```python
from build123d import *

# Parameters (mm, degrees)
SKETCH1_R                  = 1.5
BOSS_EXTRUDE1_DEPTH        = 2.54
BOSS_EXTRUDE3_DEPTH        = 15
SKETCH5_R                  = 1.5
CUT_EXTRUDE1_DEPTH         = 12.7
CHAMFER1_SIZE              = 2.54
CHAMFER1_SIZE_2            = 4.399409051
CUT_EXTRUDE5_DEPTH         = 36.401142437
CHAMFER1_OF_MIRROR1_SIZE   = 4.399409051
CHAMFER1_OF_MIRROR1_SIZE_2 = 2.54


with BuildPart() as part:
    # Sketch1 → Boss-Extrude1 (new body)
    with BuildSketch(Plane(origin=(0, 0, 0), x_dir=(1, 0, 0), z_dir=(0, 1, 0))):
        with BuildLine():
            Line((-2.46, 6.35), (20.4, 6.35))
            ThreePointArc((20.4, 6.35), (22.196051224, 5.606051224), (22.94, 3.81))
            Line((22.94, 3.81), (22.94, -3.81))
            ThreePointArc((22.94, -3.81), (22.196051224, -5.606051224), (20.4, -6.35))
            Line((20.4, -6.35), (-2.46, -6.35))
            ThreePointArc((-2.46, -6.35), (-4.256051224, -5.606051224), (-5, -3.81))
            Line((-5, -3.81), (-5, 3.81))
            ThreePointArc((-5, 3.81), (-4.256051224, 5.606051224), (-2.46, 6.35))
        make_face()
        with Locations(Location((-1.19, -2.88414655, 0), (0, 0, 270))):
            Circle(SKETCH1_R, mode=Mode.SUBTRACT)
        with Locations(Location((8.81, -2.88414655, 0), (0, 0, 270))):
            Circle(SKETCH1_R, mode=Mode.SUBTRACT)
        with Locations(Location((18.81, -2.88414655, 0), (0, 0, 270))):
            Circle(SKETCH1_R, mode=Mode.SUBTRACT)
    boss_extrude1 = extrude(amount=BOSS_EXTRUDE1_DEPTH)

    # Sketch3 → Boss-Extrude3 (add)
    with BuildSketch(Plane(origin=(0, 2.54, 0), x_dir=(1, 0, 0), z_dir=(0, 1, 0))):
        with BuildLine():
            Line((-5, 2.54), (22.94, 2.54))
            Line((22.94, 2.54), (22.94, 3.81))
            Line((22.94, 3.81), (22.94, 19.207931679))
            ThreePointArc((22.94, 19.207931679), (22.305, 20.307783942), (21.035, 20.307783942))
            Line((21.035, 20.307783942), (-3.73, 6.009704526))
            ThreePointArc((-3.73, 6.009704526), (-4.659704526, 5.08), (-5, 3.81))
            Line((-5, 3.81), (-5, 2.54))
        make_face()
    boss_extrude3 = extrude(amount=BOSS_EXTRUDE3_DEPTH)

    # Sketch5 → Cut-Extrude1 (cut)
    with BuildSketch(Plane(origin=(-5.860422493, 0, -4.779704526), x_dir=(0.8660254037844379, 0, -0.5000000000000014), z_dir=(0.5000000000000013, 0, 0.8660254037844378))):
        with Locations(Location((6.758079416, 6.35, 0), (0, 0, 180))):
            Circle(SKETCH5_R)
        with Locations(Location((26.758079416, 6.35, 0), (0, 0, 180))):
            Circle(SKETCH5_R)
    cut_extrude1 = extrude(amount=CUT_EXTRUDE1_DEPTH, mode=Mode.SUBTRACT)

    # Chamfer1
    # the kernel refuses this chamfer: 4.399409051, 2.54 mm, written as the material it adds along each edge
    with BuildSketch(Plane(origin=(-5, 2.54, -2.54), x_dir=(0, -0.057893862402671366, 0.9983227437537925), z_dir=(1, 0, 0))) as chamfer1_piece_1_section:
        Polygon((CHAMFER1_SIZE * 0.998322743754, -CHAMFER1_SIZE * 0.0578938624027), (-CHAMFER1_SIZE_2 * 0.0578938624056, -CHAMFER1_SIZE_2 * 0.998322743805), (0, 0), align=None)
    chamfer1_piece_1 = extrude(amount=27.94, mode=Mode.PRIVATE)
    chamfer1_piece_1 = chamfer1_piece_1 - Plane(origin=(5.060500306, 6.35, 0.619729795), x_dir=(-0.8660254037844379, 0, 0.5000000000000014), z_dir=(-0.5000000000000014, 0, -0.8660254037844379)) * Cylinder(1.5, 74, mode=Mode.PRIVATE)
    add(chamfer1_piece_1)

    # Sketch11 → Cut-Extrude5 (cut, symmetric)
    with BuildSketch(Plane(origin=(0, 17.54, 0), x_dir=(1, 0, 0), z_dir=(0, 1, 0))):
        Polygon((3.153238686, 9.983744234), (4.423238686, 7.784039708), (15.421761314, 14.134039708), (14.151761314, 16.333744234), align=None)
    cut_extrude5 = extrude(amount=CUT_EXTRUDE5_DEPTH, both=True, mode=Mode.SUBTRACT)

    # Mirror1: Boss-Extrude1, Boss-Extrude3, Cut-Extrude1, Cut-Extrude5 across plane
    add(boss_extrude1.mirror(Plane.XY.offset(2.88414655)))
    add(boss_extrude3.mirror(Plane.XY.offset(2.88414655)))
    add(cut_extrude1.mirror(Plane.XY.offset(2.88414655)), mode=Mode.SUBTRACT)
    add(cut_extrude5.mirror(Plane.XY.offset(2.88414655)), mode=Mode.SUBTRACT)

    # Chamfer1 of Mirror1
    # the kernel refuses this chamfer: 4.399409051, 2.54 mm, written as the material it adds along each edge
    with BuildSketch(Plane(origin=(-5, 2.54, 8.308293101), x_dir=(0, 0.9998132206222079, 0.019326765612700737), z_dir=(1, 0, 0))) as chamfer1_of_mirror1_piece_1_section:
        Polygon((CHAMFER1_OF_MIRROR1_SIZE * 0.999813220673, -CHAMFER1_OF_MIRROR1_SIZE * 0.0193267656137), (-CHAMFER1_OF_MIRROR1_SIZE_2 * 0.0193267656127, -CHAMFER1_OF_MIRROR1_SIZE_2 * 0.999813220622), (0, 0), align=None)
    chamfer1_of_mirror1_piece_1 = extrude(amount=27.94, mode=Mode.PRIVATE)
    chamfer1_of_mirror1_piece_1 = chamfer1_of_mirror1_piece_1 - Plane(origin=(5.060500238, 6.35, 5.148563423), x_dir=(-0.8660254037844379, 0, -0.5000000000000014), z_dir=(-0.5000000000000014, 0, 0.8660254037844379)) * Cylinder(1.5, 74, mode=Mode.PRIVATE)
    add(chamfer1_of_mirror1_piece_1)


solid = part.part
```
Geometry: final body of the model. Coordinates: model frame, mm. A direction names the side the tool comes from. Round coordinates to 2 decimals unless told otherwise and drop trailing zeros. Order: outer loops, then holes, each group sorted by start corner. A loop starts at its lowest first (then second) coordinate and runs counter-clockwise, first axis right, second up. Notation, with made-up numbers: (-1, 76.5) -> (14, 76.5) arc R22 cw to (14, 98.5) -> close; hole circle Ø4 at (19.5, 68). An arc over 180 degrees is marked (long way). Use one line per item in the form item = value.
(1) First-contact query: pin 1 Ø5 at (x, z) = (13.5, 18.5) entering from -Y; pin 2 Ø2 at (x, y) = (11.5, 14) entering from -Z; pin 3 Ø6 at (x, y) = (0.5, 8.5) entering from -Z. Flat tips, straight axial feed; report the tip coordinate or a pass-through.
Results list:
pin_1 = 2.54
pin_2 = -12.45
pin_3 = -9.98
(2) Section B-B on x = 8.81. Return loops of the section in (y, z), and give its area (3 significant figures).
Results list:
outline = (0, -6.35) -> (2.54, -6.35) -> (2.54, -10.32) -> (17.54, -10.32) -> (17.54, -2.54) -> (6.94, -2.54) -> (2.54, 0) -> (2.54, 1.38) -> (0, 1.38) -> close; (0, 4.38) -> (2.54, 4.38) -> (2.54, 5.77) -> (6.94, 8.31) -> (17.54, 8.31) -> (17.54, 16.09) -> (2.54, 16.09) -> (2.54, 12.12) -> (0, 12.12) -> close
area = 284 mm^2
(3) Ray query, probe 1 along Z at (x, y) = (-1.19, 1.65); probe 2 along Y at (x, z) = (9.5, 0.5); probe 3 along Z at (x, y) = (17.5, 15.5). Return the intervals inside material, ascending. Write a range as [from, to].
Results list:
probe_1 = [-6.35, 1.38], [4.38, 12.12]
probe_2 = [0, 2.54]
probe_3 = [-18.27, -2.54], [8.31, 24.04]
(4) Draft query along X for faces 6 (the face through (10.3, 1.3, 2.7)), 7 (the face through (-0.24, 9.935, 13.793)), 8 (the face through (22.18, 1.25, 11.39)). Return one class per face: pulls with the +X half, pulls with the -X half, needs draft (parallel to the pull), parting line crosses it, or undercut.
Results list:
face_6 = undercut
face_7 = pulls with the -X half
face_8 = pulls with the +X half
(5) Section A-A on y = 15.25. Return loops of the section in (x, z) (3 decimals), and give its area (3 significant figures).
Results list:
outline = (-5, -3.81) arc R2.54 ccw to (-3.73, -6.01) -> (3.153, -9.984) -> (4.423, -7.784) -> (15.422, -14.134) -> (14.152, -16.334) -> (21.035, -20.308) arc R1.27 ccw to (22.94, -19.208) -> (22.94, -2.54) -> (-5, -2.54) -> close; (-5, 8.308) -> (22.94, 8.308) -> (22.94, 24.976) arc R1.27 ccw to (21.035, 26.076) -> (14.152, 22.102) -> (15.422, 19.902) -> (4.423, 13.552) -> (3.153, 15.752) -> (-3.73, 11.778) arc R2.54 ccw to (-5, 9.578) -> close
area = 536 mm^2
(6) Access query for faces 1 (the face through (9, 1, -6.35)), 2 (the face through (14.796, 10.145, -15.218)), 3 (the face through (9, 0, 1)), 4 (the face through (22.2, 1.3, -5.6)), 5 (the face through (9, 12, -2.54)). Directions: +Z, -Z, +X, -X, +Y, -Y. A direction counts if a zero-diameter tool reaches every point of the face in a straight line with its end or side. Return the directions, or none.
Results list:
face_1 = -Z, +X, -X, -Y
face_2 = -X, +Y, -Y
face_3 = +Z, -Z, +X, -X, -Y
face_4 = -Z, +X, -Y
face_5 = +X, -X, +Y
